Geometry: see drawing. Coordinates: mm, zero at the bounding-box minimum. A direction names the side the tool comes from. Round coordinates to 2 decimals unless told otherwise and drop trailing zeros. Write each loop counter-clockwise with the first axis right and the second up, starting at its lowest first coordinate (ties: lowest second). Pieces come first, ordered by that corner, then holes. Notation, with made-up numbers: M -38,45.5 L -32,45.5 A19 cw -32,63.5 Z; hole C 43,25.25 d2. An arc over 180 degrees is marked long. Use one line per item in the form item = value. Start each with the question number.
Item 1: Ray query, probe 1 along X at (y, z) = (7.75, 3). Return the intervals inside material, ascending.
Item 2: Section query A-A (y = 10). Return loops of the section in (x, z), and give its area (3 significant figures).
Item 3: Section query C-C (y = 16.75). Return loops of the section in (x, z), and give its area (3 significant figures).
Item 4: Reachability of the marked faces 1, 2 and 3 from +Z, -Z, +X, -X, +Y, -Y: full face, straight path, thin tool, end or side. Return the list, or none.
Item 5: Section query B-B (z = 30). Return loops of the section in (x, y).
Item 6: Section query D-D (z = 12). Return loops of the section in (x, y).
Item 7: Pin query (flat end, axial travel): pin 1 Ø4 at (y, z) = (10, 24) entering from +X; pin 2 Ø10 at (y, z) = (10.5, 12.5) entering from -X. Return the tip coordinate at first contact, or that it passes through.
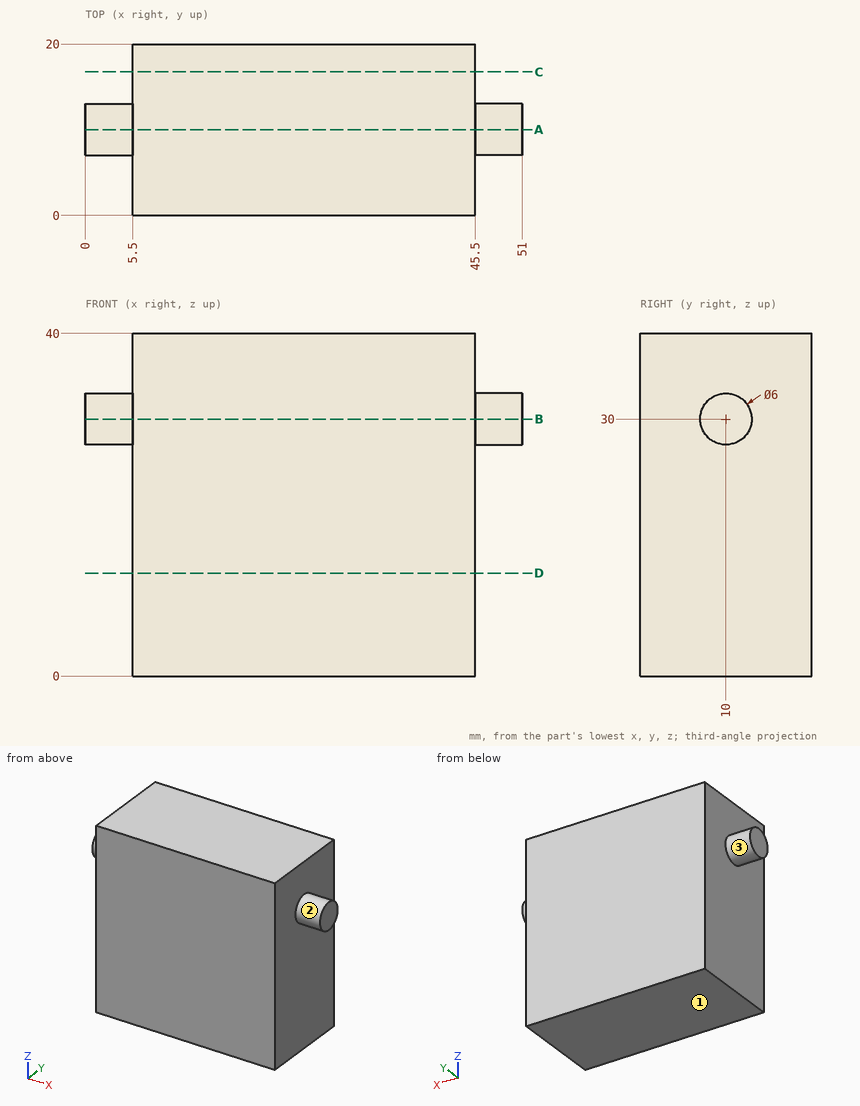
Working result:
q1.probe_1 = 5.5 to 45.5
q2.outline = M 0,27 L 5.5,27 L 5.5,0 L 45.5,0 L 45.5,27 L 51,27 L 51,33 L 45.5,33 L 45.5,40 L 5.5,40 L 5.5,33 L 0,33 Z
q2.area = 1,670 mm²
q3.outline = M 5.5,0 L 45.5,0 L 45.5,40 L 5.5,40 Z
q3.area = 1,600 mm²
q4.face_1 = -Z, +X, -X, +Y, -Y
q4.face_2 = +X
q4.face_3 = -X
q5.outline = M 0,7 L 5.5,7 L 5.5,0 L 45.5,0 L 45.5,7 L 51,7 L 51,13 L 45.5,13 L 45.5,20 L 5.5,20 L 5.5,13 L 0,13 Z
q6.outline = M 5.5,0 L 45.5,0 L 45.5,20 L 5.5,20 Z
q7.pin_1 = 45.5
q7.pin_2 = 5.5
